Design review of the part built by this model. Coordinates are the model's own, in mm. Face numbers are marked on the shaded views. Coordinates: 2 decimals unless noted, no trailing zeros. Loops run counter-clockwise (first coordinate to the right, second up) from the corner with the lowest first, then second, coordinate; pieces in that order, holes last. Notation, with made-up numbers: M -37.75,-25 L 7.25,-25 A23 cw 7.25,3 Z; hole C 74,84 d10. An arc over 180 degrees is marked long. One line per item, written item: value.
```python
from build123d import *

# Parameters (mm, degrees)
SK_BLOCK_W       = 32
SK_BLOCK_H       = 33
BLOCK_DEPTH      = 26
SK_PITCH_BORE_R  = 4
PITCH_BORE_DEPTH = 40
SK_ROLL_BORE_R   = 4
ROLL_BORE_DEPTH  = 40


with BuildPart() as part:
    # SK_Block → Block (new body)
    with BuildSketch(Plane.XY.offset(-13)):
        Rectangle(SK_BLOCK_W, SK_BLOCK_H)
    extrude(amount=BLOCK_DEPTH)

    # SK_Pitch_Bore → Pitch_Bore (cut)
    with BuildSketch(Plane(origin=(0, -20, 0), x_dir=(1, 0, 0), z_dir=(0, 1, 0))):
        with Locations(Location((0, 0, 0), (0, 0, 90))):
            Circle(SK_PITCH_BORE_R)
    extrude(amount=PITCH_BORE_DEPTH, mode=Mode.SUBTRACT)

    # SK_Roll_Bore → Roll_Bore (cut)
    with BuildSketch(Plane(origin=(-20, 0, 0), x_dir=(0, 0, -1), z_dir=(1, 0, 0))):
        Circle(SK_ROLL_BORE_R)
    extrude(amount=ROLL_BORE_DEPTH, mode=Mode.SUBTRACT)


solid = part.part
```
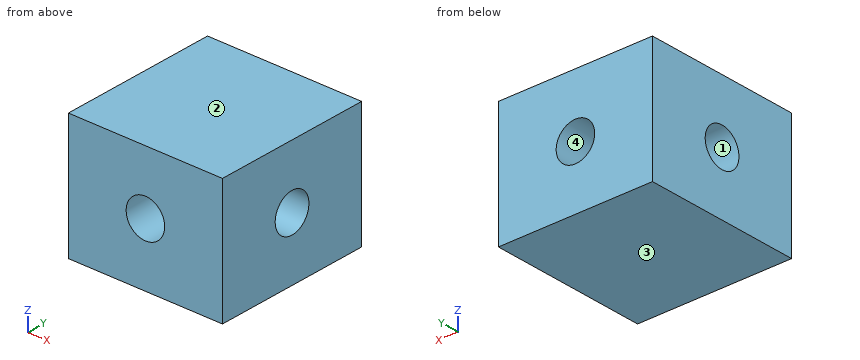
(1) We need section B-B on y = 7. State the section outline as (x, z) points, then the cut area to 3 significant figures.
Reply:
outline: M -16,-13 L 16,-13 L 16,13 L -16,13 Z; hole C 0,0 d8
area: 782 mm2
(2) We need section D-D on y = 2. State the section outline as (x, z) points.
Reply:
outline: M -16,-13 L 16,-13 L 16,-3.46 L 2,-3.46 A4 cw -2,-3.46 L -16,-3.46 Z; M -16,3.46 L -2,3.46 A4 cw 2,3.46 L 16,3.46 L 16,13 L -16,13 Z
(3) We need section A-A on z = 0. State the section outline as (x, y) points, then the cut area to 3 significant figures.
Reply:
outline: M -16,-16.5 L -4,-16.5 L -4,-4 L -16,-4 Z; M -16,4 L -4,4 L -4,16.5 L -16,16.5 Z; M 4,-16.5 L 16,-16.5 L 16,-4 L 4,-4 Z; M 4,4 L 16,4 L 16,16.5 L 4,16.5 Z
area: 600 mm2
(4) Mouldability with a two-part tool opening along Z and no side actions: class the marked faces 1, 2, 3 and 4 as released by +Z, released by -Z, zero draft, split by the parting line, or undercut.
Reply:
face 1: undercut
face 2: released by +Z
face 3: released by -Z
face 4: undercut
(5) To check wall thickness, follow line 1 along Y through (x, z) = (5, -0.25); line 2 along Z through (x, y) = (-5.5, 0); line 3 along X through (y, z) = (-8.75, 0). State the ranges of each line that lie inside material, in increasing order. Write a range as [from, to].
Reply:
line 1: y = [-16.5, -3.99], [3.99, 16.5]
line 2: z = [-13, -4], [4, 13]
line 3: x = [-16, -4], [4, 16]
(6) We need section C-C on x = -2. State the section outline as (y, z) points, then the cut area to 3 significant figures.
Reply:
outline: M -16.5,-13 L 16.5,-13 L 16.5,-3.46 L 2,-3.46 A4 cw -2,-3.46 L -16.5,-3.46 Z; M -16.5,3.46 L -2,3.46 A4 cw 2,3.46 L 16.5,3.46 L 16.5,13 L -16.5,13 Z
area: 626 mm2
